```python
from build123d import *

# Parameters (mm, degrees)
SKETCH1_W               = 22
SKETCH1_H               = 6
BOSS_EXTRUDE1_DEPTH     = 23
BOSS_EXTRUDE2_DEPTH     = 23
BOSS_EXTRUDE3_DEPTH     = 23
CUT_EXTRUDE1_DEPTH      = 24
SKETCH5_W               = 20
SKETCH5_H               = 2
BOSS_EXTRUDE4_DEPTH     = 45
SKETCH6_W               = 1
SKETCH6_H               = 2
BOSS_EXTRUDE5_DEPTH     = 20
BOSS_EXTRUDE6_DEPTH     = 23
FILLET1_R               = 0.6
BOSS_EXTRUDE7_DEPTH     = 23
FILLET2_R               = 0.9
SKETCH10_W              = 21.8
SKETCH10_H              = 5
CUT_EXTRUDE2_DEPTH      = 23
CUT_EXTRUDE2_DEPTH_BACK = 24
SKETCH11_R              = 1.725
CUT_EXTRUDE3_DEPTH      = 18.25
SKETCH12_R              = 3
CUT_EXTRUDE4_DEPTH      = 2


with BuildPart() as part:
    # Sketch1 → Boss-Extrude1 (new body)
    with BuildSketch(Plane(origin=(0, 0, 0), x_dir=(1, 0, 0), z_dir=(0, 1, 0))):
        Rectangle(SKETCH1_W, SKETCH1_H)
    extrude(amount=BOSS_EXTRUDE1_DEPTH)

    # Sketch2 → Boss-Extrude2 (add)
    with BuildSketch(Plane(origin=(0, 23, 0), x_dir=(1, 0, 0), z_dir=(0, 1, 0))):
        with BuildLine():
            Line((-11, 3), (-7.342667591, 3))
            ThreePointArc((-7.342667591, 3), (-31.353026246, 1.686257741), (-8.610829915, -6.125))
            Line((-8.610829915, -6.125), (-11.641918828, -4.375))
            ThreePointArc((-11.641918828, -4.375), (-27.936683546, 0.758729989), (-11, 3))
        make_face()
        with BuildLine():
            Line((11.641918828, -4.375), (8.610829915, -6.125))
            ThreePointArc((8.610829915, -6.125), (31.353026246, 1.686257741), (7.342667591, 3))
            Line((7.342667591, 3), (11, 3))
            ThreePointArc((11, 3), (27.936683546, 0.758729989), (11.641918828, -4.375))
        make_face()
    extrude(amount=-BOSS_EXTRUDE2_DEPTH)

    # Sketch3 → Boss-Extrude3 (add)
    with BuildSketch(Plane(origin=(0, 23, 0), x_dir=(1, 0, 0), z_dir=(0, 1, 0))):
        with BuildLine():
            Line((-19.219641111, 12.25), (19.219641111, 12.25))
            ThreePointArc((19.219641111, 12.25), (11.692606503, 9.66469089), (7.342667591, 3))
            Line((7.342667591, 3), (-7.342667591, 3))
            ThreePointArc((-7.342667591, 3), (-11.692606503, 9.66469089), (-19.219641111, 12.25))
        make_face()
    extrude(amount=-BOSS_EXTRUDE3_DEPTH)

    # Sketch8 → Cut-Extrude1 (cut, through all)
    with BuildSketch(Plane.XZ):
        Polygon((11, 2.863163975), (7.215123909, -3.692433715), (3.837624834, -1.742433715), (6.575670216, 3), (11, 3), align=None)
        Polygon((-6.575670216, 3), (-11, 3), (-11, 2.863163975), (-7.215123909, -3.692433715), (-3.837624834, -1.742433715), align=None)
    extrude(amount=-CUT_EXTRUDE1_DEPTH, mode=Mode.SUBTRACT)

    # Sketch5 → Boss-Extrude4 (add)
    with BuildSketch(Plane(origin=(0, 23, 0), x_dir=(1, 0, 0), z_dir=(0, 1, 0))):
        with Locations((0, 13.25)):
            Rectangle(SKETCH5_W, SKETCH5_H)
    extrude(amount=-BOSS_EXTRUDE4_DEPTH)

    # Sketch6 → Boss-Extrude5 (add)
    with BuildSketch(Plane.ZY.offset(10)):
        with Locations((-11.75, -21)):
            Rectangle(SKETCH6_W, SKETCH6_H)
        Polygon((-11.25, -20), (-11.25, -22), (-9.25, -22), (-9.25, -1), (-11.25, -1), align=None)
    extrude(amount=-BOSS_EXTRUDE5_DEPTH)

    # Sketch9 → Boss-Extrude6 (add)
    with BuildSketch(Plane.XZ):
        Polygon((4.160829915, -1.582626094), (8.610829915, 6.125), (11.641918828, 4.375), (7.191918828, -3.332626094), align=None)
        Polygon((-7.191918828, -3.332626094), (-4.160829915, -1.582626094), (-8.610829915, 6.125), (-11.641918828, 4.375), align=None)
    extrude(amount=-BOSS_EXTRUDE6_DEPTH)

    # Fillet1
    fillet1_edges = [part.edges().sort_by_distance(p)[0] for p in [
        (11, 11.5, 2.863163975),
        (6.575670216, 11.5, 3),
        (-6.575670216, 11.5, 3),
        (-11, 11.5, 2.863163975),
    ]]
    fillet(fillet1_edges, radius=FILLET1_R)

    # Sketch7 → Boss-Extrude7 (add)
    with BuildSketch(Plane(origin=(0, 23, 0), x_dir=(1, 0, 0), z_dir=(0, 1, 0))):
        with BuildLine():
            Line((10, 14.25), (19.219641111, 14.25))
            ThreePointArc((19.219641111, 14.25), (31.560503115, -7.125), (6.878779107, -7.125))
            Line((6.878779107, -7.125), (8.610829915, -6.125))
            ThreePointArc((8.610829915, -6.125), (29.828452308, -6.125), (19.219641111, 12.25))
            Line((19.219641111, 12.25), (10, 12.25))
            Line((10, 12.25), (10, 14.25))
        make_face()
        with BuildLine():
            Line((-8.610829915, -6.125), (-6.878779107, -7.125))
            ThreePointArc((-6.878779107, -7.125), (-31.560503115, -7.125), (-19.219641111, 14.25))
            Line((-19.219641111, 14.25), (-10, 14.25))
            Line((-10, 14.25), (-10, 12.25))
            Line((-10, 12.25), (-19.219641111, 12.25))
            ThreePointArc((-19.219641111, 12.25), (-29.828452308, -6.125), (-8.610829915, -6.125))
        make_face()
    extrude(amount=-BOSS_EXTRUDE7_DEPTH)

    # Fillet2
    fillet2_edges = [part.edges().sort_by_distance(p)[0] for p in [
        (0, -22, -9.25),
        (-8.610829915, 11.5, 6.125),
        (6.878779107, 11.5, 7.125),
        (10, 0, -13.25),
        (-6.878779107, 11.5, 7.125),
        (-10, 0, -13.25),
        (8.610829915, 11.5, 6.125),
        (0, -22, -14.25),
    ]]
    fillet(fillet2_edges, radius=FILLET2_R)

    # Sketch10 → Cut-Extrude2 (cut, two sides)
    with BuildSketch(Plane.XZ) as cut_extrude2_sk:
        with Locations((0, -11.75)):
            Rectangle(SKETCH10_W, SKETCH10_H)
    extrude(amount=CUT_EXTRUDE2_DEPTH, mode=Mode.SUBTRACT)
    extrude(cut_extrude2_sk.sketch, amount=-CUT_EXTRUDE2_DEPTH_BACK, mode=Mode.SUBTRACT)

    # Sketch11 → Cut-Extrude3 (cut, through all)
    with BuildSketch(Plane.XY.offset(3)):
        with Locations((0, 5)):
            Circle(SKETCH11_R)
        with Locations((0, 18)):
            Circle(SKETCH11_R)
    extrude(amount=-CUT_EXTRUDE3_DEPTH, mode=Mode.SUBTRACT)

    # Sketch12 → Cut-Extrude4 (cut)
    with BuildSketch(Plane.XY.offset(3)):
        with Locations((0, 5)):
            Circle(SKETCH12_R)
        with Locations((0, 18)):
            Circle(SKETCH12_R)
    extrude(amount=-CUT_EXTRUDE4_DEPTH, mode=Mode.SUBTRACT)


solid = part.part
```
Geometry: final body of the model. Coordinates: model frame, mm. A direction names the side the tool comes from. Round coordinates to 2 decimals unless told otherwise and drop trailing zeros. Order: outer loops, then holes, each group sorted by start corner. A loop starts at its lowest first (then second) coordinate and runs counter-clockwise, first axis right, second up. Notation, with made-up numbers: (63.5, 62) -> (88.5, 62) arc R33 ccw to (88.5, 92) -> close; hole circle Ø11 at (-26, -4). An arc over 180 degrees is marked (long way). Use CSV: the item, a comma, the result in double quotes. Start each with the question number.
1) Set-up query: faces 3 (the face through (5.7, 11.34, -2.47)), 4 (the face through (0, 16, 1)), 5 (the face through (0, 11, 3)). Return all of +Z, -Z, +X, -X, +Y, -Y with unobstructed straight access to the full face (end or side cutting, diameter ignored); none if empty.
2) Section A-A (z = 0). State how many separate pieces and enclosed holes the cut face has, and give its area (3 significant figures).
3) Section B-B (x = 0). Return the cut outline in (y, z) (3 decimals), and give its area (3 significant figures).
4) First-contact query: pin 1 Ø1.5 at (y, z) = (8.5, 5) entering from -X; pin 2 Ø3 at (y, z) = (14, 10.5) entering from +X; pin 3 Ø5.5 at (x, y) = (-0.5, 16) entering from +Z; pin 4 Ø8 at (y, z) = (3, 4) entering from -X. Flat tips, straight axial feed; report the tip coordinate or a pass-through.
5) Material intervals for line 1 along Y through (x, z) = (0, -6) (3 decimals); line 2 along X through (y, z) = (15, 4); line 3 along X through (y, z) = (6, 2.5), sorted ascending. Write a range as from..to.
6) Draft query along X for faces 1 (the face through (15, 12, -14.25)), 2 (the face through (-7.26, 11.34, 7.23)). Return one class per face: +X half, -X half, draft (parallel to the pull), parting line (faces both ways), or undercut.
7) Section D-D (x = 18). Return the cut outline in (y, z).
Returned:
1,face 3,"+Y, -Y"
1,face 4,"+Z"
1,face 5,"+Z, +Y, -Y"
2,separate pieces,"7"
2,enclosed holes,"2"
2,area,"719 mm²"
3,outline,"(0, -9.25) -> (3.275, -9.25) -> (3.275, 1) -> (2, 1) -> (2, 3) -> (0, 3) -> close; (6.725, -9.25) -> (16.275, -9.25) -> (16.275, 1) -> (15, 1) -> (15, 3) -> (8, 3) -> (8, 1) -> (6.725, 1) -> close; (19.725, -9.25) -> (23, -9.25) -> (23, 3) -> (21, 3) -> (21, 1) -> (19.725, 1) -> close"
3,area,"187 mm²"
4,pin 1,"stops at x = -32.82"
4,pin 2,"stops at x = 30.27"
4,pin 3,"stops at z = 3"
4,pin 4,"stops at x = -33.47"
5,line 1,"y = 0..3.275, 6.725..16.275, 19.725..23"
5,line 2,"x = -32.9..-27, -11.43..-7.38, 7.38..11.43, 27..32.9"
5,line 3,"x = -33.25..-27.6, -10.56..-6.52, -6.13..-2.83, 2.83..6.13, 6.52..10.56, 27.6..33.25"
6,face 1,"draft"
6,face 2,"undercut"
7,outline,"(0, -14.25) -> (23, -14.25) -> (23, -8.66) -> (0, -8.66) -> close; (0, 8.66) -> (23, 8.66) -> (23, 14.2) -> (0, 14.2) -> close"
